Autodesk Inventor part; units mm, degrees
ref_plane "YZ Plane" through (0, 0, 0) normal (1, 0, 0) x (0, 1, 0)
ref_plane "XZ Plane" through (0, 0, 0) normal (0, 1, 0) x (-1, 0, 0)
ref_plane "XY Plane" through (0, 0, 0) normal (0, 0, 1) x (1, 0, 0)
sketch "스케치1" plane through (0, 0, 0) normal (0, 0, 1) x (1, 0, 0)
  circle A0 centre (0, 0) radius 0.9
  circle A1 centre (0, 0) radius 1.6
  line L0 (-0.5568, 1.5) -> (-3.5568, 1.5)
  line L1 (-3.5568, 1.5) -> (-3.5568, -1.5)
  line L2 (-3.5568, -1.5) -> (-0.5568, -1.5)
  circle A2 centre (0, 0) radius 1.25
  point P0 (-0.2784, -0.75)
  point P1 (-0.2784, 0.75)
  point P2 (-3.5568, 0)
  dimension "d0" = 1.8
  dimension "d3" = 3.2
  dimension "d6" = 3
  dimension "d7" = 3
  dimension "d10" = 2.5
extrude "돌출1" add sketch "스케치1" along normal mid plane 16 contours A0
extrude "돌출2" add sketch "스케치1" along normal mid plane 12.8 contours A1 | A2
extrude "돌출3" add sketch "스케치1" along normal mid plane 16 contours A1 L2 L1 L0
extrude "돌출4" [suppressed]
sketch "스케치2" plane through (-3.5568, -0.75, 4) normal (-1, 0, 0) x (0, 0, 1)
  line L0 (4, 2.25) -> (4, 0.75)
  line L1 (-12, 2.25) -> (4, 2.25)
  line L2 (-12, 0.75) -> (-12, 2.25)
  arc A0 (4, 2.25) -> (-12, 2.25) centre (-4, 2.25) ccw
  line L3 (-12, 2.25) -> (-12, -19.75)
  line L4 (-12, -19.75) -> (4, -19.75)
  line L5 (4, -19.75) -> (4, 2.25)
  point P0 (-4, 0.75)
  dimension "d15" = 22
  dimension "d52" = 8
  dimension "d53" = 16
  dimension "d54" = 8
extrude "돌출5" add sketch "스케치2" along normal blind 1
sketch "스케치4" plane through (-3.5568, -0.75, 4) normal (1, 0, 0) x (0, 0, -1)
  line L0 (3.25, 5) -> (4.75, 5)
  line L1 (4.75, 5) -> (4.75, 6.5)
  line L2 (4.75, 6.5) -> (3.25, 6.5)
  line L3 (3.25, 6.5) -> (3.25, 5)
  line L4 (3.25, 5) -> (4.75, 6.5) construction
  line L5 (4.75, 5) -> (3.25, 6.5) construction
  line L6 (2, 5) -> (3, 5)
  line L7 (3, 5) -> (3, 6.5)
  line L8 (3, 6.5) -> (2, 6.5)
  line L9 (2, 6.5) -> (2, 5)
  line L10 (2, 5) -> (3, 6.5) construction
  line L11 (3, 5) -> (2, 6.5) construction
  line L12 (6, 5) -> (5, 5)
  line L13 (5, 5) -> (5, 6.5)
  line L14 (5, 6.5) -> (6, 6.5)
  line L15 (6, 6.5) -> (6, 5)
  line L16 (6, 5) -> (5, 6.5) construction
  line L17 (5, 5) -> (6, 6.5) construction
  point P0 (4, 0.75)
  point P1 (4, 5.75)
  point P2 (2.5, 5.75)
  point P3 (5.5, 5.75)
  dimension "d26" = 1.5
  dimension "d27" = 1.5
  dimension "d28" = 1
  dimension "d29" = 1
  dimension "d30" = 1.5
  dimension "d31" = 3
  dimension "d32" = 5
extrude "돌출7" add sketch "스케치4" along normal blind 1.5 contours L9 L8 L7 L6 | L12 L13 L14 L15
sketch "스케치5" plane through (0, 0, 0) normal (0, 0, 1) x (1, 0, 0)
  circle A0 centre (-2.8068, 5) radius 0.5
  circle A1 centre (-2.8068, 5) radius 0.4
  line L0 (-2.8068, 4.5) -> (0.1861, 4.4792)
  line L1 (0.1861, 4.4792) -> (0.1932, 5.5)
  line L2 (0.1932, 5.5) -> (-2.8068, 5.5)
  line L3 (-3.5568, 4.25) -> (-2.0568, 4.25)
  point P0 (0, 0)
  point P1 (-2.8068, 4.25)
  dimension "d35" = 5
  dimension "d36" = 1
  dimension "d37" = 0.8
  dimension "d49" = 3
extrude "돌출8" cut sketch "스케치5" along normal through all both and the other way through all contours A0 | A1
extrude "돌출9" [suppressed]
extrude "돌출10" [suppressed]
sketch "스케치6" plane through (0, 0, 8) normal (0, 0, 1) x (1, 0, 0)
  line L0 (-4.5568, -20.5) -> (-4.5568, 1.5)
  line L1 (-3.5568, -20.5) -> (-4.5568, -20.5)
  line L2 (-3.5568, -20.5) -> (-3.5568, -1.5)
  line L3 (-4.5568, -19.1) -> (-3.5568, -16.6)
  dimension "d55" = 1.4
  dimension "d61" = 3.9
extrude "돌출11" cut sketch "스케치6" against normal through all
fillet "모깎기9" radius 0.5 11 edges at (-4.5568, 9.5, 0) (-4.5568, -8.8, -8) (-4.5568, -8.8, 8) (-3.5568, 5.75, 1.5) (-2.0568, 5.75, 1.5) (-2.0568, 4.25, 1.5) (-3.5568, 4.25, 1.5) (-3.5568, 4.25, -1.5) (-3.5568, 5.75, -1.5) (-2.0568, 5.75, -1.5) (-2.0568, 4.25, -1.5)
fillet "모깎기10" radius 2 1 edges at (-3.5568, -16.6, 0)
fillet "모깎기11" radius 0.5 4 edges at (-0.5568, 1.5, 7.2) (-0.5568, -1.5, 7.2) (-0.5568, 1.5, -7.2) (-0.5568, -1.5, -7.2)
fillet "모깎기12" radius 1.7 2 edges at (-3.5568, -1.5, 0) (-3.5568, 1.5, 0)
equation "\"d29\" = d28"
properties part number "집게 이동"
Geometry: final body of the model. Coordinates: model frame, mm. A direction names the side the tool comes from. Give positions to 0.01 mm unless a question says otherwise; leave off trailing zeros. Order: outer loops, then holes, each group sorted by start corner. A loop starts at its lowest first (then second) coordinate and runs counter-clockwise, first axis right, second up. Notation, with made-up numbers: (-35.5, 80.25) - (13.5, 80.25) arc R25 ccw to (13.5, 92.25) - close; hole circle Ø1 at (-13, 43.25). An arc over 180 degrees is marked (long way). Use CSV: the item, a comma, the result in double quotes.
1. Access query for faces 4 (the face through (0.86, 0.27, -7.19)), 5 (the face through (-1, 1.5, 0)), 6 (the face through (-1, 1, 6.4)). Directions: +Z, -Z, +X, -X, +Y, -Y. A direction counts if a zero-diameter tool reaches every point of the face in a straight line with its end or side. Return the directions, or none.
Answers below:
face 4,"-Z"
face 5,"+Z, -Z, +Y"
face 6,"+Z"
2. Section query D-D (y = -2.5). Output: boundary loops of the cut face in (x, z), plus the area to 3 significant figures.
Answers below:
outline,"(-4.56, -7.5) arc R0.5 ccw to (-4.06, -8) - (-3.41, -8) - (-3.41, 8) - (-4.06, 8) arc R0.5 ccw to (-4.56, 7.5) - close"
area,"18.3 mm2"
3. Material intervals for line 1 along Y through (x, z) = (-0.75, -4.75); line 2 along Z through (x, y) = (-3.5, 4.5); line 3 along X through (y, z) = (1.25, -4.75), sorted ascending. Write a range as from..to.
Answers below:
line 1,"-1.5..1.5"
line 2,"-2..-1, 1..2"
line 3,"-4.56..1"
4. Section query A-A (z = 0). Output: boundary loops of the cut face in (x, y).
Answers below:
outline,"(-4.56, -19.1) - (-3.7, -16.96) arc R2 ccw to (-3.56, -16.21) - (-3.56, -3.2) arc R1.7 cw to (-1.86, -1.5) - (-0.56, -1.5) arc R1.6 ccw (long way) to (-0.56, 1.5) - (-1.86, 1.5) arc R1.7 cw to (-3.56, 3.2) - (-3.56, 9.5) - (-4.06, 9.5) arc R0.5 ccw to (-4.56, 9) - close"
5. Section query C-C (y = -11.5). Output: boundary loops of the cut face in (x, z).
Answers below:
outline,"(-4.56, -7.5) arc R0.5 ccw to (-4.06, -8) - (-3.56, -8) - (-3.56, 8) - (-4.06, 8) arc R0.5 ccw to (-4.56, 7.5) - close"
6. Mould query, pull axis Y, two halves, no side actions, for faces 1 (the face through (-2.33, 5.15, 1.51)), 2 (the face through (-3.046, -1.985, 0.112)), 3 (the face through (-3.8, 9.5, -0.1)). Classes: +Y half, -Y half, draft (parallel to the pull), parting line (faces both ways), or undercut.
Answers below:
face 1,"undercut"
face 2,"-Y half"
face 3,"+Y half"
7. Contact query for flat-ended pins moving along their axis: pin 1 (7 mm diameter, centred on y = 6, z = 0, fed in from +X); pin 2 (5 mm diameter, centred on y = -7, z = 2, fed in from +X); pin 3 (1 mm diameter, centred on x = -1.5, z = 3.5, fed in from +Y). Output: stop coordinate, or through.
Answers below:
pin 1,"x = -2.06"
pin 2,"x = -3.56"
pin 3,"y = 1.51"
8. Section query B-B (x = 0). Output: boundary loops of the cut face in (y, z), plus the area to 3 significant figures.
Answers below:
outline,"(-1.6, -6.4) - (-0.9, -6.4) - (-0.9, -8) - (0.9, -8) - (0.9, -6.4) - (1.6, -6.4) - (1.6, 6.4) - (0.9, 6.4) - (0.9, 8) - (-0.9, 8) - (-0.9, 6.4) - (-1.6, 6.4) - close"
area,"46.7 mm2"
